Part print with two shaded views. Sizes in mm from the minimum x, y, z corner. Round coordinates to 2 decimals unless told otherwise and drop trailing zeros. Loops run counter-clockwise (first coordinate to the right, second up) from the corner with the lowest first, then second, coordinate; pieces in that order, holes last.
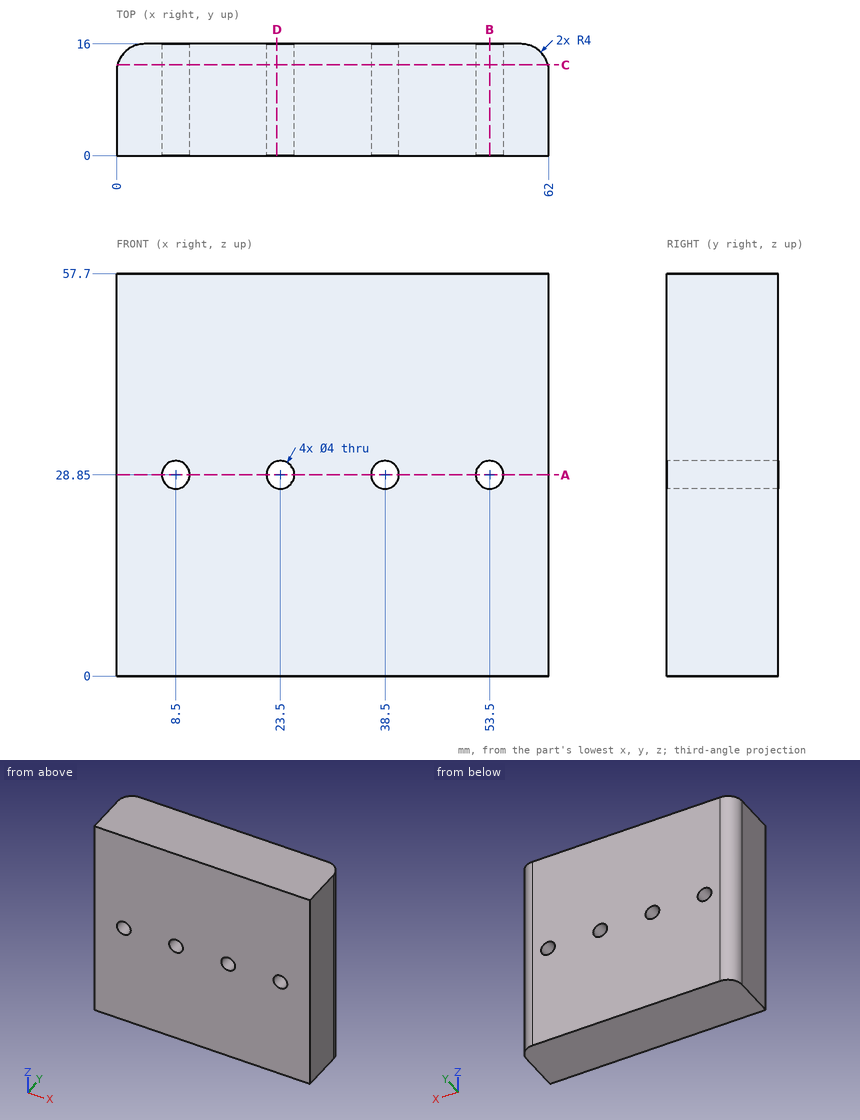
Item 1: Cut at C-C (y = 13). List the corners of the cut face in (x, z).
Verdict:
outline: (0.13, 0) - (61.87, 0) - (61.87, 57.7) - (0.13, 57.7) - close; hole circle Ø4 at (8.5, 28.85); hole circle Ø4 at (23.5, 28.85); hole circle Ø4 at (38.5, 28.85); hole circle Ø4 at (53.5, 28.85)
Item 2: Wall check: L1, parallel to Z at x = 8.5, y = 10.5; L2, parallel to Z at x = 55, y = 4.25; L3, parallel to Y at x = 59.5, z = 25. Give the ranges that are in metal, low to high.
Verdict:
L1: z = 0 to 26.85, 30.85 to 57.7
L2: z = 0 to 27.53, 30.17 to 57.7
L3: y = 0 to 15.71
Item 3: Flat gauge pin, fed straight in: P1, Ø1.5, axis at y = 14, z = 28, coming from the -X side. Where does the tip first touch, or does it go through?
Verdict:
P1: stops at x = 0.2
Item 4: Cut at A-A (z = 28.85). List the corners of the cut face in (x, y).
Verdict:
outline: (0, 0) - (6.5, 0) - (6.5, 16) - (4, 16) arc R4 ccw to (0, 12) - close; (10.5, 0) - (21.5, 0) - (21.5, 16) - (10.5, 16) - close; (25.5, 0) - (36.5, 0) - (36.5, 16) - (25.5, 16) - close; (40.5, 0) - (51.5, 0) - (51.5, 16) - (40.5, 16) - close; (55.5, 0) - (62, 0) - (62, 12) arc R4 ccw to (58, 16) - (55.5, 16) - close
Item 5: Cut at B-B (x = 53.5). List the corners of the cut face in (y, z), plus the area to 3 significant figures.
Verdict:
outline: (0, 0) - (16, 0) - (16, 26.85) - (0, 26.85) - close; (0, 30.85) - (16, 30.85) - (16, 57.7) - (0, 57.7) - close
area: 859 mm2
Item 6: Cut at D-D (x = 23). List the corners of the cut face in (y, z).
Verdict:
outline: (0, 0) - (16, 0) - (16, 26.91) - (0, 26.91) - close; (0, 30.79) - (16, 30.79) - (16, 57.7) - (0, 57.7) - close
